The listing builds one solid part. Answer for the finished solid, in the listing's coordinates (mm). Face numbers are marked on the shaded views. A direction names the side the tool comes from. Give positions to 0.01 mm unless a question says otherwise; leave off trailing zeros. Order: outer loops, then holes, each group sorted by start corner. A loop starts at its lowest first (then second) coordinate and runs counter-clockwise, first axis right, second up. Notation, with made-up numbers: (84, 31) - (108, 31) arc R18 cw to (108, 57) - close; hole circle Ø8 at (28.5, -13.75). An arc over 180 degrees is marked (long way). Answer as a JSON object with one key per item and string values. Group by question number.
Q1. Consider line 1 (X direction, y = 1.05, z = 5); line 2 (X direction, y = 1.8, z = -5); line 3 (Y direction, x = -27, z = -5.5). Determine where each line is inside the solid, lowest interval first.
Q2. A cutting plane is placed at A-A, the plane z = -23. Give the vertices of the cut face in (x, y).
Q3. A cutting plane is placed at D-D, the plane z = -2.5. Give the vertices of the cut face in (x, y), and give its area (3 significant figures).
Q4. A cutting plane is placed at C-C, the plane x = 0. Give the vertices of the cut face in (y, z), and give its area (3 significant figures).
Q5. Given pin 1 (8 mm diameter, centred on x = -17, y = 3.5, fed in from -Z); pin 2 (1.5 mm diameter, centred on x = 45, y = 1.5, fed in from -Z); pin 3 (6 mm diameter, centred on x = -22.5, y = 13, fed in from +Z); pin 4 (12 mm diameter, centred on y = 13.5, z = 12.5, fed in from +X), each flat-ended and moving along its own axis, determine where each tip first touches the part or whether it passes through.
Q6. A cutting plane is placed at B-B, the plane x = 47. Give the vertices of the cut face in (y, z).
Q7. For the marked faces 4, 5 and 6, determine the directions among +Z, -Z, +X, -X, +Y, -Y from which every point of the face is accessible in a straight line to the end or side of a thin tool.
Q8. The mould has two halves that part along X. Classify the marked faces 1, 2 and 3: released by +X, released by -X, zero draft, split by the parting line, or undercut.
from build123d import *

# Parameters (mm, degrees)
BOSS_EXTRUDE1_DEPTH = 27
BOSS_EXTRUDE2_DEPTH = 2
BOSS_EXTRUDE3_DEPTH = 1
SKETCH4_R           = 1.5
CUT_EXTRUDE1_DEPTH  = 42.701318924
SKETCH5_W           = 27.460607986
SKETCH5_H           = 18
BOSS_EXTRUDE4_DEPTH = 3
SKETCH6_R           = 1.5
SKETCH6_R_2         = 6
CUT_EXTRUDE2_DEPTH  = 59.129166517
BOSS_EXTRUDE5_DEPTH = 10
SKETCH8_W           = 6
SKETCH8_H           = 1.5
BOSS_EXTRUDE6_DEPTH = 20


with BuildPart() as part:
    # Sketch1 → Boss-Extrude1 (new, symmetric)
    with BuildSketch(Plane.XY):
        with BuildLine():
            Line((-31, 3), (-23.539392014, 3))
            ThreePointArc((-23.539392014, 3), (-14, 10), (-4.460607986, 3))
            Line((-4.460607986, 3), (4.460607986, 3))
            ThreePointArc((4.460607986, 3), (14, 10), (23.539392014, 3))
            Line((23.539392014, 3), (31, 3))
            Line((31, 3), (31, 0))
            Line((31, 0), (21.5, 0))
            ThreePointArc((21.5, 0), (14, 7.5), (6.5, 0))
            Line((6.5, 0), (-6.5, 0))
            ThreePointArc((-6.5, 0), (-14, 7.5), (-21.5, 0))
            Line((-21.5, 0), (-31, 0))
            Line((-31, 0), (-31, 3))
        make_face()
    extrude(amount=BOSS_EXTRUDE1_DEPTH, both=True)

    # Sketch2 → Boss-Extrude2 (add)
    with BuildSketch(Plane.XY.offset(27)):
        with BuildLine():
            Line((-22, 0), (-21, 0))
            ThreePointArc((-21, 0), (-14, 7), (-7, 0))
            Line((-7, 0), (-6, 0))
            ThreePointArc((-6, 0), (-14, 8), (-22, 0))
        make_face()
        with BuildLine():
            Line((21, 0), (22, 0))
            ThreePointArc((22, 0), (14, 8), (6, 0))
            Line((6, 0), (7, 0))
            ThreePointArc((7, 0), (14, 7), (21, 0))
        make_face()
    boss_extrude2 = extrude(amount=-BOSS_EXTRUDE2_DEPTH)

    # Mirror1: Boss-Extrude2 across plane
    add(boss_extrude2.mirror(Plane.XY))

    # Sketch3 → Boss-Extrude3 (add, symmetric)
    with BuildSketch(Plane.XY):
        with BuildLine():
            Line((-22, 0), (-21, 0))
            ThreePointArc((-21, 0), (-14, 7), (-7, 0))
            Line((-7, 0), (-6, 0))
            ThreePointArc((-6, 0), (-14, 8), (-22, 0))
        make_face()
        with BuildLine():
            Line((6, 0), (7, 0))
            ThreePointArc((7, 0), (14, 7), (21, 0))
            Line((21, 0), (22, 0))
            ThreePointArc((22, 0), (14, 8), (6, 0))
        make_face()
    extrude(amount=BOSS_EXTRUDE3_DEPTH, both=True)

    # Sketch4 → Cut-Extrude1 (cut, through all)
    with BuildSketch(Plane(origin=(0, 3, 0), x_dir=(1, 0, 0), z_dir=(0, 1, 0))):
        with Locations(Location((-27, 23, 0), (0, 0, 270))):
            Circle(SKETCH4_R)
        with Locations(Location((-27, -23, 0), (0, 0, 270))):
            Circle(SKETCH4_R)
        with Locations(Location((27, -23, 0), (0, 0, 270))):
            Circle(SKETCH4_R)
        with Locations(Location((27, 23, 0), (0, 0, 270))):
            Circle(SKETCH4_R)
        with Locations(Location((0, 0, 0), (0, 0, 270))):
            Circle(SKETCH4_R)
    extrude(amount=-CUT_EXTRUDE1_DEPTH, mode=Mode.SUBTRACT)

    # Sketch5 → Boss-Extrude4 (add)
    with BuildSketch(Plane(origin=(0, 3, 0), x_dir=(1, 0, 0), z_dir=(0, 1, 0))):
        with Locations((37.269696007, 0)):
            Rectangle(SKETCH5_W, SKETCH5_H)
    extrude(amount=-BOSS_EXTRUDE4_DEPTH)

    # Sketch6 → Cut-Extrude2 (cut, through all)
    with BuildSketch(Plane(origin=(0, 3, 0), x_dir=(1, 0, 0), z_dir=(0, 1, 0))):
        with Locations(Location((47, 5, 0), (0, 0, 270))):
            Circle(SKETCH6_R)
        with Locations(Location((47, -5, 0), (0, 0, 270))):
            Circle(SKETCH6_R)
        with Locations(Location((27, -5, 0), (0, 0, 270))):
            Circle(SKETCH6_R)
        with Locations(Location((27, 5, 0), (0, 0, 270))):
            Circle(SKETCH6_R)
        with Locations(Location((37, 0, 0), (0, 0, 270))):
            Circle(SKETCH6_R_2)
    extrude(amount=-CUT_EXTRUDE2_DEPTH, mode=Mode.SUBTRACT)

    # Sketch7 → Boss-Extrude5 (add, symmetric)
    with BuildSketch(Plane.XY):
        with BuildLine():
            Line((-27.269696007, 3), (-23.539392014, 3))
            ThreePointArc((-23.539392014, 3), (-20.416966951, 7.669585071), (-15.269696007, 9.919066088))
            Line((-15.269696007, 9.919066088), (-15.269696007, 20.5))
            Line((-15.269696007, 20.5), (-27.269696007, 20.5))
            Line((-27.269696007, 20.5), (-27.269696007, 3))
        make_face()
    extrude(amount=BOSS_EXTRUDE5_DEPTH, both=True)

    # Sketch8 → Boss-Extrude6 (add)
    with BuildSketch(Plane(origin=(0, 0, -10), x_dir=(-1, 0, 0), z_dir=(0, 0, -1))):
        with Locations((18.269696007, 21.25)):
            Rectangle(SKETCH8_W, SKETCH8_H)
    extrude(amount=-BOSS_EXTRUDE6_DEPTH)


solid = part.part
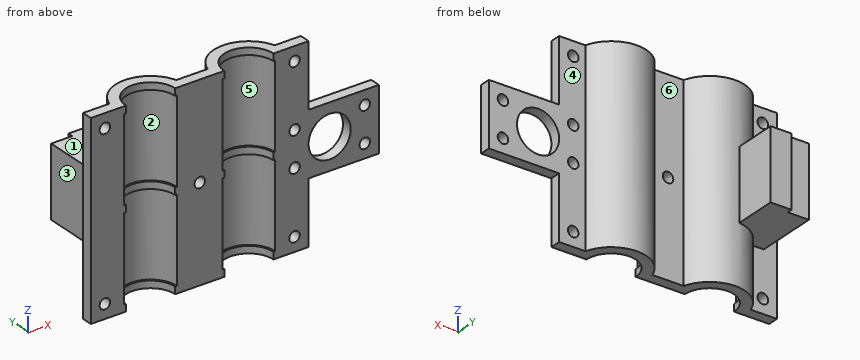
Reply:
{
 "1": {"line 1": "x = -31 to -21.43, -6.57 to 6.57, 21.43 to 25.5, 28.5 to 33.68, 40.32 to 45.5, 48.5 to 51", "line 2": "x = -31 to -21.28, -6.72 to 6.72, 21.28 to 25.5, 28.5 to 33.68, 40.32 to 45.5, 48.5 to 51", "line 3": "y = 0 to 20.5"},
 "2": {"outline": "(-31, 0) - (-28.5, 0) - (-28.5, 3) - (-31, 3) - close; (-25.5, 0) - (-21.5, 0) arc R7.5 cw to (-6.5, 0) - (6.5, 0) arc R7.5 cw to (21.5, 0) - (25.5, 0) - (25.5, 3) - (23.54, 3) arc R10 ccw to (4.46, 3) - (-4.46, 3) arc R10 ccw to (-23.54, 3) - (-25.5, 3) - close; (28.5, 0) - (31, 0) - (31, 3) - (28.5, 3) - close"},
 "3": {"outline": "(-31, 0) - (-21.5, 0) arc R7.5 cw to (-6.5, 0) - (6.5, 0) arc R7.5 cw to (21.5, 0) - (31.55, 0) - (31.55, 3) - (23.54, 3) arc R10 ccw to (4.46, 3) - (-4.46, 3) arc R10 ccw to (-15.27, 9.92) - (-15.27, 22) - (-21.27, 22) - (-21.27, 20.5) - (-27.27, 20.5) - (-27.27, 3) - (-31, 3) - close; (42.45, 0) - (51, 0) - (51, 3) - (42.45, 3) - close", "area": "411 mm^2"},
 "4": {"outline": "(0, -27) - (3, -27) - (3, -1.5) - (0, -1.5) - close; (0, 1.5) - (3, 1.5) - (3, 27) - (0, 27) - close", "area": "153 mm^2"},
 "5": {"pin 1": "stops at z = -27", "pin 2": "stops at z = -9", "pin 3": "stops at z = 10", "pin 4": "stops at x = 20.61"},
 "6": {"outline": "(0, -9) - (3, -9) - (3, -6.5) - (0, -6.5) - close; (0, -3.5) - (3, -3.5) - (3, 3.5) - (0, 3.5) - close; (0, 6.5) - (3, 6.5) - (3, 9) - (0, 9) - close"},
 "7": {"face 4": "+Z, -Z, +X, +Y", "face 5": "-Y", "face 6": "+Z, -Z, +Y"},
 "8": {"face 1": "zero draft", "face 2": "undercut", "face 3": "released by -X"}
}
